```python
from build123d import *

# Parameters (mm, degrees)
BOSS_EXTRUDE1_DEPTH     = 9
SKETCH2_W               = 5.6
SKETCH2_H               = 2
CUT_EXTRUDE1_DEPTH      = 8.3
CUT_EXTRUDE2_DEPTH      = 22.914607001
CUT_EXTRUDE5_REACH      = 23.915
CUT_EXTRUDE5_END_RADIUS = 1.65
SKETCH16_R              = 1.5
FILLET2_R               = 1
SKETCH6_R               = 1.6
CUT_EXTRUDE3_DEPTH      = 22.914607049
CUT_EXTRUDE4_DEPTH      = 3
FILLET3_R               = 1
FILLET1_R               = 2


with BuildPart() as part:
    # Sketch1 → Boss-Extrude1 (new body)
    with BuildSketch(Plane(origin=(0, 0, 0), x_dir=(1, 0, 0), z_dir=(0, 1, 0))):
        Polygon((10.5, 10.5), (17, 4), (17, 0), (0, 0), align=None)
    extrude(amount=BOSS_EXTRUDE1_DEPTH)

    # Sketch2 → Cut-Extrude1 (cut)
    with BuildSketch(Plane(origin=(0, 9, 0), x_dir=(1, 0, 0), z_dir=(0, 1, 0))):
        with Locations((12, 2.5)):
            Rectangle(SKETCH2_W, SKETCH2_H)
    extrude(amount=-CUT_EXTRUDE1_DEPTH, mode=Mode.SUBTRACT)

    # Sketch4 → Cut-Extrude2 (cut, through all)
    with BuildSketch(Plane.XY):
        with BuildLine():
            ThreePointArc((12.49446871, 1.925833333), (12, 5.15), (11.50553129, 1.925833333))
            ThreePointArc((11.50553129, 1.925833333), (12, 1.5), (12.49446871, 1.925833333))
        make_face()
    extrude(amount=-CUT_EXTRUDE2_DEPTH, mode=Mode.SUBTRACT)

    # Cut-Extrude5: up to this cylinder (the profile starts outside it)
    cut_extrude5_end = Plane(origin=(12, 3.5, -3), z_dir=(0, 0, 1)) * Cylinder(CUT_EXTRUDE5_END_RADIUS, 52.13, mode=Mode.PRIVATE)
    # Sketch16 → Cut-Extrude5 (cut, up to the surface)
    with BuildSketch(Plane(origin=(0, 9, 0), x_dir=(1, 0, 0), z_dir=(0, 1, 0)), mode=Mode.PRIVATE) as cut_extrude5_sk1:
        with Locations((12, 3)):
            Circle(SKETCH16_R)
    cut_extrude5_tool1 = extrude(cut_extrude5_sk1.sketch, amount=-CUT_EXTRUDE5_REACH, mode=Mode.PRIVATE) - cut_extrude5_end
    add(cut_extrude5_tool1.solids().sort_by_distance((12, 9, -3))[0], mode=Mode.SUBTRACT)

    # Fillet2
    fillet2_edges = [part.edges().sort_by_distance(p)[0] for p in [
        (14.8, 9, -2.5),
        (9.2, 9, -2.5),
    ]]
    fillet(fillet2_edges, radius=FILLET2_R)

    # Sketch6 → Cut-Extrude3 (cut, through all)
    with BuildSketch(Plane(origin=(0, 9, 0), x_dir=(1, 0, 0), z_dir=(0, 1, 0))):
        with Locations((4.5, 4.5)):
            Circle(SKETCH6_R)
    extrude(amount=-CUT_EXTRUDE3_DEPTH, mode=Mode.SUBTRACT)

    # Sketch9 → Cut-Extrude4 (cut)
    with BuildSketch(Plane.XZ):
        Polygon((7.511458693, -5.306917925), (6.704540769, -2.295459231), (3.693082075, -1.488541307), (1.488541307, -3.693082075), (2.295459231, -6.704540769), (5.306917925, -7.511458693), align=None)
    extrude(amount=-CUT_EXTRUDE4_DEPTH, mode=Mode.SUBTRACT)

    # Fillet3
    fillet3_edges = [part.edges().sort_by_distance(p)[0] for p in [
        (6.960323501, 0, -5.858053117),
        (7.107999731, 0, -3.801188578),
        (5.198811422, 0, -1.892000269),
        (3.141946883, 0, -2.039676499),
    ]]
    fillet(fillet3_edges, radius=FILLET3_R)

    # Mirror1: part across plane


with BuildPart() as part_1:
    add(part.part)
    add(part.part.mirror(Plane(origin=(0, 9, 0), x_dir=(-0.7071067811865432, 0, 0.7071067811865518), z_dir=(0.707106781186552, 0, 0.7071067811865431))))

    # Fillet1
    fillet1_edges = [part_1.edges().sort_by_distance(p)[0] for p in [
        (0, 4.5, 0),
    ]]
    fillet(fillet1_edges, radius=FILLET1_R)


solid = part_1.part
```
CAD build for the part. Positions are in the model's coordinates, mm. A direction names the side the tool comes from. Give positions to 0.01 mm unless a question says otherwise; leave off trailing zeros. Loops run counter-clockwise (first coordinate to the right, second up) from the corner with the lowest first, then second, coordinate; pieces in that order, holes last. Notation, with made-up numbers: (79, 28.25) -> (84, 28.25) arc R20 cw to (84, 48.25) -> close; hole circle Ø2 at (30.25, -1.5). An arc over 180 degrees is marked (long way). Use a Markdown table: item, result.
1. Slice it at A-A (y = 3.75). Give the number of separate pieces and of enclosed holes in the cut face, plus the area to 3 significant figures.
Check result:
| item | result |
|---|---|
| separate pieces | 3 |
| enclosed holes | 1 |
| area | 128 mm^2 |
2. Slice it at C-C (z = -14). List the corners of the cut face in (x, y).
Check result:
| item | result |
|---|---|
| outline | (0, 0) -> (7, 0) -> (7, 9) -> (3.5, 9) -> (3.5, 0.7) -> (1.5, 0.7) -> (1.5, 9) -> (0, 9) -> close |
3. Slice it at B-B (z = -12.25). List the corners of the cut face in (x, y), plus the area to 3 significant figures.
Check result:
| item | result |
|---|---|
| outline | (0, 0) -> (8.75, 0) -> (8.75, 1.57) -> (3.5, 1.57) -> (3.5, 0.7) -> (1.5, 0.7) -> (1.5, 1.57) -> (0, 1.57) -> close; (0, 5.13) -> (1.5, 5.13) -> (1.5, 9) -> (0, 9) -> close; (4.48, 5.13) -> (8.75, 5.13) -> (8.75, 9) -> (4.48, 9) -> close |
| area | 34.3 mm^2 |
4. Slice it at D-D (y = 8.25). List the corners of the cut face in (x, z), plus the area to 3 significant figures.
Check result:
| item | result |
|---|---|
| outline | (0, -17) -> (4, -17) -> (17, -4) -> (17, 0) -> (2, 0) arc R2 ccw to (0, -2) -> close; hole (1.5, -14.83) -> (3.5, -14.83) -> (3.5, -13.41) arc R1.5 ccw to (3.5, -10.59) -> (3.5, -9.17) -> (1.5, -9.17) -> close; hole circle Ø3.2 at (4.5, -4.5); hole (9.17, -3.5) -> (10.59, -3.5) arc R1.5 ccw to (13.41, -3.5) -> (14.83, -3.5) -> (14.83, -1.5) -> (9.17, -1.5) -> close |
| area | 169 mm^2 |
5. Which spindle directions (+Z, -Z, +X, -X, +Y, -Y) get a long thin tool onto all of the face, cutting with end or side? Do faces 1 (the flat face through (0, 4, -10)), 2 (the flat face through (12, 6, -1.5)), 3 (the cylindrical face through (1.594, 0.285, -5.248)). Say none if no direction does.
Check result:
| item | result |
|---|---|
| face 1 | +Z, -Z, -X, +Y, -Y |
| face 2 | +Y |
| face 3 | -Y |
6. Mould opens along Z. For faces 4 (the flat face through (11, 5, -10)), 5 (the cylindrical face through (5.92, 6.04, -5.24)), 6 (the cylindrical face through (0.6, 4.56, -0.57)), 7 (the flat face through (9, 0, -7)) say: pulls with the +Z half, pulls with the -Z half, needs draft (parallel to the pull), parting line crosses it, or undercut.
Check result:
| item | result |
|---|---|
| face 4 | pulls with the -Z half |
| face 5 | undercut |
| face 6 | pulls with the +Z half |
| face 7 | needs draft |
7. Wall check: L1, parallel to Y at x = 0.8, z = -12; L2, parallel to X at y = 2, z = -6.5; L3, parallel to X at y = 3.5, z = -10.25. Give the ranges that are in metal, low to high. Write a range as [from, to].
Check result:
| item | result |
|---|---|
| L1 | y = [0, 1.5], [5.15, 9] |
| L2 | x = [0, 2.24], [6.32, 11.31], [12.69, 14.5] |
| L3 | x = [0, 1.5], [3.5, 10.35] |
8. Flat gauge pins, fed straight in: pin 1 (2.5 mm diameter, centred on x = 12, y = 3.5, fed in from +Z) (3 decimals); pin 2 (1.5 mm diameter, centred on y = 4, z = -7.5, fed in from +X); pin 3 (2.5 mm diameter, centred on y = 6, z = -13.5, fed in from +X); pin 4 (2 mm diameter, centred on x = 12, z = -3, fed in from +Y). Where does each tip first touch, or does it go through?
Check result:
| item | result |
|---|---|
| pin 1 | passes through |
| pin 2 | stops at x = 14.25 |
| pin 3 | stops at x = 8.75 |
| pin 4 | stops at y = 2.1 |
